```python
from build123d import *

# Parameters (mm, degrees)
SALIENTE_EXTRUIR1_DEPTH = 6
CROQUIS4_W              = 5
CROQUIS4_H              = 50
SALIENTE_EXTRUIR4_DEPTH = 80
CROQUIS5_R              = 8
CROQUIS5_R_2            = 7.5
CORTAR_EXTRUIR1_DEPTH   = 80


with BuildPart() as part:
    # Croquis1 → Saliente-Extruir1 (new body)
    with BuildSketch(Plane(origin=(0, 0, 0), x_dir=(1, 0, 0), z_dir=(0, 1, 0))):
        with BuildLine():
            Line((-9.5, 4.5), (-9.5, 0))
            Line((-9.5, 0), (-4.5, 0))
            ThreePointArc((-4.5, 0), (-3.181980515, 3.181980515), (0, 4.5))
            Line((0, 4.5), (-9.5, 4.5))
        make_face()
        with BuildLine():
            Line((-4.5, 0), (-9.5, 0))
            Line((-9.5, 0), (-9.5, -4.5))
            Line((-9.5, -4.5), (0, -4.5))
            ThreePointArc((0, -4.5), (-3.181980515, -3.181980515), (-4.5, 0))
        make_face()
        with BuildLine():
            ThreePointArc((0, 4.5), (-3.181980515, 3.181980515), (-4.5, 0))
            Line((-4.5, 0), (-2.5, 0))
            ThreePointArc((-2.5, 0), (-2.236067977, 1.118033989), (-1.5, 2))
            Line((-1.5, 2), (-1.5, 3.446675318))
            Line((-1.5, 3.446675318), (0, 3.446675318))
            Line((0, 3.446675318), (0, 4.5))
        make_face()
        with BuildLine():
            Line((-2.5, 0), (-4.5, 0))
            ThreePointArc((-4.5, 0), (-3.181980515, -3.181980515), (0, -4.5))
            Line((0, -4.5), (0, -3.446675318))
            Line((0, -3.446675318), (-1.5, -3.446675318))
            Line((-1.5, -3.446675318), (-1.5, -2))
            ThreePointArc((-1.5, -2), (-2.236067977, -1.118033989), (-2.5, 0))
        make_face()
        with BuildLine():
            ThreePointArc((-1.5, 2), (-2.236067977, 1.118033989), (-2.5, 0))
            Line((-2.5, 0), (-1.5, 0))
            Line((-1.5, 0), (-1.5, 2))
        make_face()
        with BuildLine():
            Line((-1.5, 0), (-2.5, 0))
            ThreePointArc((-2.5, 0), (-2.236067977, -1.118033989), (-1.5, -2))
            Line((-1.5, -2), (-1.5, 0))
        make_face()
        with BuildLine():
            Line((-1.5, 3.446675318), (-1.5, 2))
            ThreePointArc((-1.5, 2), (-0.790569415, 2.371708245), (0, 2.5))
            Line((0, 2.5), (0, 3.446675318))
            Line((0, 3.446675318), (-1.5, 3.446675318))
        make_face()
        with BuildLine():
            Line((1.5, 3.446675318), (0, 3.446675318))
            Line((0, 3.446675318), (0, 2.5))
            ThreePointArc((0, 2.5), (0.790569415, 2.371708245), (1.5, 2))
            Line((1.5, 2), (1.5, 3.446675318))
        make_face()
        with BuildLine():
            ThreePointArc((0, -2.5), (-0.790569415, -2.371708245), (-1.5, -2))
            Line((-1.5, -2), (-1.5, -3.446675318))
            Line((-1.5, -3.446675318), (0, -3.446675318))
            Line((0, -3.446675318), (0, -2.5))
        make_face()
        with BuildLine():
            Line((0, -2.5), (0, -3.446675318))
            Line((0, -3.446675318), (1.5, -3.446675318))
            Line((1.5, -3.446675318), (1.5, -2))
            ThreePointArc((1.5, -2), (0.790569415, -2.371708245), (0, -2.5))
        make_face()
        with BuildLine():
            ThreePointArc((1.5, -2), (2.236067977, -1.118033989), (2.5, 0))
            Line((2.5, 0), (1.5, 0))
            Line((1.5, 0), (1.5, -2))
        make_face()
        with BuildLine():
            Line((1.5, 0), (2.5, 0))
            ThreePointArc((2.5, 0), (2.236067977, 1.118033989), (1.5, 2))
            Line((1.5, 2), (1.5, 0))
        make_face()
        with BuildLine():
            ThreePointArc((4.5, 0), (3.181980515, 3.181980515), (0, 4.5))
            Line((0, 4.5), (0, 3.446675318))
            Line((0, 3.446675318), (1.5, 3.446675318))
            Line((1.5, 3.446675318), (1.5, 2))
            ThreePointArc((1.5, 2), (2.236067977, 1.118033989), (2.5, 0))
            Line((2.5, 0), (4.5, 0))
        make_face()
        with BuildLine():
            Line((0, -3.446675318), (0, -4.5))
            ThreePointArc((0, -4.5), (3.181980515, -3.181980515), (4.5, 0))
            Line((4.5, 0), (2.5, 0))
            ThreePointArc((2.5, 0), (2.236067977, -1.118033989), (1.5, -2))
            Line((1.5, -2), (1.5, -3.446675318))
            Line((1.5, -3.446675318), (0, -3.446675318))
        make_face()
    extrude(amount=SALIENTE_EXTRUIR1_DEPTH)

    # Croquis4 → Saliente-Extruir4 (add)
    with BuildSketch(Plane(origin=(0, 6, 0), x_dir=(1, 0, 0), z_dir=(0, 1, 0))):
        with Locations((-7, 0)):
            Rectangle(CROQUIS4_W, CROQUIS4_H)
    extrude(amount=SALIENTE_EXTRUIR4_DEPTH)

    # Croquis5 → Cortar-Extruir1 (cut)
    with BuildSketch(Plane.ZY.offset(9.5)):
        with Locations((-13, 26)):
            Circle(CROQUIS5_R)
        with Locations((13, 26)):
            Circle(CROQUIS5_R)
        with Locations((0, 69)):
            Circle(CROQUIS5_R_2)
    extrude(amount=-CORTAR_EXTRUIR1_DEPTH, mode=Mode.SUBTRACT)


solid = part.part
```
Design review of the part built by this model. Coordinates are the model's own, in mm. A direction names the side the tool comes from. Give positions to 0.01 mm unless a question says otherwise; leave off trailing zeros. Order: outer loops, then holes, each group sorted by start corner. A loop starts at its lowest first (then second) coordinate and runs counter-clockwise, first axis right, second up. Notation, with made-up numbers: (9, -0.5) - (66, -0.5) arc R28 cw to (66, 17.5) - close; hole circle Ø9 at (-22, -39). An arc over 180 degrees is marked (long way). Use a Markdown table: item, result. Add a question column.
(1) Add section C-C on x = -5.5. Give the boundary of the cut face in (y, z), then the cut area to 3 significant figures.
(2) Mouldability with a two-part tool opening along Z and no side actions: class faces 4 (the face through (-7, 45, -25)), 5 (the face through (-2, 6, 0)), 6 (the face through (-1.5, 3, 0)), 7 (the face through (-5, 3, 4.5)) as +Z half, -Z half, draft (parallel to the pull), parting line (faces both ways), or undercut.
(3) Clearance check with flat-ended pins moving along their axes: P1, Ø13, axis at y = 26, z = 13, coming from the +X side; P2, Ø5.5, axis at x = -7.5, z = -10.5, coming from the -Y side; P3, Ø7, axis at x = 1.5, z = 1, coming from the +Y side; P4, Ø1, axis at y = 63.5, z = 20, coming from the +X side. State where each tip first meets the part, or that it passes through.
(4) Add section D-D on y = 26. Give the boundary of the cut face in (x, z).
(5) Machinability: for faces 1 (the face through (-5, 3, -4.5)), 2 (the face through (1.5, 3, 0)), 3 (the face through (-7, 6, 15)), which of the approach directions +Z, -Z, +X, -X, +Y, -Y give a long, thin tool a straight path to every point of the face, cutting with its end or side? Answer none if there is none.
(6) Add section A-A on z = 13. Give the boundary of the cut face in (x, y).
(7) Wall thickness on probe 1 along Y at (x, z) = (-8.05, 13); probe 2 along Y at (x, z) = (-5.5, 0); probe 3 along X at (y, z) = (32.5, -21.5): over which ranges is each line inside the solid? List them lowest first. Write a range as [from, to].
(8) Add section B-B on y = 69. Give the boundary of the cut face in (x, z), then the cut area to 3 significant figures.
Report:
| question | item | result |
|---|---|---|
| 1 | outline | (0, -4.5) - (6, -4.5) - (6, -25) - (86, -25) - (86, 25) - (6, 25) - (6, 4.5) - (0, 4.5) - close; hole circle Ø16 at (26, -13); hole circle Ø16 at (26, 13); hole circle Ø15 at (69, 0) |
| 1 | area | 3,480 mm² |
| 2 | face 4 | -Z half |
| 2 | face 5 | draft |
| 2 | face 6 | undercut |
| 2 | face 7 | +Z half |
| 3 | P1 | passes through |
| 3 | P2 | stops at y = 6 |
| 3 | P3 | stops at y = 6 |
| 3 | P4 | stops at x = -4.5 |
| 4 | outline | (-9.5, -25) - (-4.5, -25) - (-4.5, -21) - (-9.5, -21) - close; (-9.5, -5) - (-4.5, -5) - (-4.5, 5) - (-9.5, 5) - close; (-9.5, 21) - (-4.5, 21) - (-4.5, 25) - (-9.5, 25) - close |
| 5 | face 1 | -Z, +X, -X, -Y |
| 5 | face 2 | +Y, -Y |
| 5 | face 3 | +Z, +X, -X, -Y |
| 6 | outline | (-9.5, 6) - (-4.5, 6) - (-4.5, 18) - (-9.5, 18) - close; (-9.5, 34) - (-4.5, 34) - (-4.5, 86) - (-9.5, 86) - close |
| 7 | probe 1 | y = [6, 18], [34, 86] |
| 7 | probe 2 | y = [0, 61.5], [76.5, 86] |
| 7 | probe 3 | x = [-9.5, -4.5] |
| 8 | outline | (-9.5, -25) - (-4.5, -25) - (-4.5, -7.5) - (-9.5, -7.5) - close; (-9.5, 7.5) - (-4.5, 7.5) - (-4.5, 25) - (-9.5, 25) - close |
| 8 | area | 175 mm² |
